Check sheet for the modelled part. Datum: model origin and axes. Units: mm. Give positions to 0.01 mm unless a question says otherwise; leave off trailing zeros.
from build123d import *

# Parameters (mm, degrees)
SKETCH1_W                      = 1219.2
SKETCH1_H                      = 1219.2
BOSS_EXTRUDE1_DEPTH            = 3.175
F_5_16_0_3125_DIAMETER_HOLE1_D = 7.9375
SKETCH5_W                      = 460.375
SKETCH5_H                      = 34.925
CUT_EXTRUDE1_DEPTH             = 863.110434124
CUT_EXTRUDE2_DEPTH             = 863.110434124
SKETCH8_W                      = 50.8
SKETCH8_H                      = 9.525
CUT_EXTRUDE3_DEPTH             = 863.110434124
SKETCH9_W                      = 298.45
SKETCH9_H                      = 3.175
CUT_EXTRUDE4_DEPTH             = 863.110434124
FILLET1_R                      = 3.175


with BuildPart() as part:
    # Sketch1 → Boss-Extrude1 (new body)
    with BuildSketch(Plane(origin=(0, 0, 0), x_dir=(1, 0, 0), z_dir=(0, 1, 0))):
        Rectangle(SKETCH1_W, SKETCH1_H)
    extrude(amount=BOSS_EXTRUDE1_DEPTH)

    # 5/16 (0.3125) Diameter Hole1 (through all)
    with Locations(Plane(origin=(0, 3.175, 0), x_dir=(1, 0, 0), z_dir=(0, 1, 0))):
        with Locations((-409.575, 377.825), (-22.225, 304.8), (22.225, 304.8), (409.575, 377.825), (-22.225, -304.8), (-409.575, -377.825), (409.575, -377.825), (22.225, -304.8)):
            Hole(F_5_16_0_3125_DIAMETER_HOLE1_D / 2)

    # Sketch5 → Cut-Extrude1 (cut, through all)
    with BuildSketch(Plane(origin=(0, 3.175, 0), x_dir=(1, 0, 0), z_dir=(0, 1, 0))):
        with Locations((-379.4125, 592.1375)):
            Rectangle(SKETCH5_W, SKETCH5_H)
        with Locations((379.4125, 592.1375)):
            Rectangle(SKETCH5_W, SKETCH5_H)
        with Locations((379.4125, -592.1375)):
            Rectangle(SKETCH5_W, SKETCH5_H)
        with Locations((-379.4125, -592.1375)):
            Rectangle(SKETCH5_W, SKETCH5_H)
    extrude(amount=-CUT_EXTRUDE1_DEPTH, mode=Mode.SUBTRACT)

    # Sketch7 → Cut-Extrude2 (cut, through all)
    with BuildSketch(Plane(origin=(0, 3.175, 0), x_dir=(1, 0, 0), z_dir=(0, 1, 0))):
        with BuildLine():
            Line((-428.625, 571.5), (-390.525, 571.5))
            ThreePointArc((-390.525, 571.5), (-384.175, 565.15), (-390.525, 558.8))
            Line((-390.525, 558.8), (-428.625, 558.8))
            ThreePointArc((-428.625, 558.8), (-434.975, 565.15), (-428.625, 571.5))
        make_face()
        with BuildLine():
            Line((-428.625, 196.85), (-390.525, 196.85))
            ThreePointArc((-390.525, 196.85), (-384.175, 190.5), (-390.525, 184.15))
            Line((-390.525, 184.15), (-428.625, 184.15))
            ThreePointArc((-428.625, 184.15), (-434.975, 190.5), (-428.625, 196.85))
        make_face()
        with BuildLine():
            Line((-38.1, 190.5), (-38.1, 152.4))
            ThreePointArc((-38.1, 152.4), (-44.45, 146.05), (-50.8, 152.4))
            Line((-50.8, 152.4), (-50.8, 190.5))
            ThreePointArc((-50.8, 190.5), (-44.45, 196.85), (-38.1, 190.5))
        make_face()
        with BuildLine():
            Line((-428.625, -571.5), (-390.525, -571.5))
            ThreePointArc((-390.525, -571.5), (-384.175, -565.15), (-390.525, -558.8))
            Line((-390.525, -558.8), (-428.625, -558.8))
            ThreePointArc((-428.625, -558.8), (-434.975, -565.15), (-428.625, -571.5))
        make_face()
        with BuildLine():
            Line((-428.625, -196.85), (-390.525, -196.85))
            ThreePointArc((-390.525, -196.85), (-384.175, -190.5), (-390.525, -184.15))
            Line((-390.525, -184.15), (-428.625, -184.15))
            ThreePointArc((-428.625, -184.15), (-434.975, -190.5), (-428.625, -196.85))
        make_face()
        with BuildLine():
            Line((-38.1, -190.5), (-38.1, -152.4))
            ThreePointArc((-38.1, -152.4), (-44.45, -146.05), (-50.8, -152.4))
            Line((-50.8, -152.4), (-50.8, -190.5))
            ThreePointArc((-50.8, -190.5), (-44.45, -196.85), (-38.1, -190.5))
        make_face()
        with BuildLine():
            Line((428.625, 571.5), (390.525, 571.5))
            ThreePointArc((390.525, 571.5), (384.175, 565.15), (390.525, 558.8))
            Line((390.525, 558.8), (428.625, 558.8))
            ThreePointArc((428.625, 558.8), (434.975, 565.15), (428.625, 571.5))
        make_face()
        with BuildLine():
            Line((428.625, 196.85), (390.525, 196.85))
            ThreePointArc((390.525, 196.85), (384.175, 190.5), (390.525, 184.15))
            Line((390.525, 184.15), (428.625, 184.15))
            ThreePointArc((428.625, 184.15), (434.975, 190.5), (428.625, 196.85))
        make_face()
        with BuildLine():
            Line((-44.45, 571.5), (44.45, 571.5))
            ThreePointArc((44.45, 571.5), (50.8, 565.15), (44.45, 558.8))
            Line((44.45, 558.8), (-44.45, 558.8))
            ThreePointArc((-44.45, 558.8), (-50.8, 565.15), (-44.45, 571.5))
        make_face()
        with BuildLine():
            Line((38.1, 190.5), (38.1, 152.4))
            ThreePointArc((38.1, 152.4), (44.45, 146.05), (50.8, 152.4))
            Line((50.8, 152.4), (50.8, 190.5))
            ThreePointArc((50.8, 190.5), (44.45, 196.85), (38.1, 190.5))
        make_face()
        with BuildLine():
            Line((428.625, -571.5), (390.525, -571.5))
            ThreePointArc((390.525, -571.5), (384.175, -565.15), (390.525, -558.8))
            Line((390.525, -558.8), (428.625, -558.8))
            ThreePointArc((428.625, -558.8), (434.975, -565.15), (428.625, -571.5))
        make_face()
        with BuildLine():
            Line((428.625, -196.85), (390.525, -196.85))
            ThreePointArc((390.525, -196.85), (384.175, -190.5), (390.525, -184.15))
            Line((390.525, -184.15), (428.625, -184.15))
            ThreePointArc((428.625, -184.15), (434.975, -190.5), (428.625, -196.85))
        make_face()
        with BuildLine():
            Line((38.1, -190.5), (38.1, -152.4))
            ThreePointArc((38.1, -152.4), (44.45, -146.05), (50.8, -152.4))
            Line((50.8, -152.4), (50.8, -190.5))
            ThreePointArc((50.8, -190.5), (44.45, -196.85), (38.1, -190.5))
        make_face()
        with BuildLine():
            Line((-44.45, -558.8), (44.45, -558.8))
            ThreePointArc((44.45, -558.8), (50.8, -565.15), (44.45, -571.5))
            Line((44.45, -571.5), (-44.45, -571.5))
            ThreePointArc((-44.45, -571.5), (-50.8, -565.15), (-44.45, -558.8))
        make_face()
    extrude(amount=-CUT_EXTRUDE2_DEPTH, mode=Mode.SUBTRACT)

    # Sketch8 → Cut-Extrude3 (cut, through all)
    with BuildSketch(Plane(origin=(0, 3.175, 0), x_dir=(1, 0, 0), z_dir=(0, 1, 0))):
        with Locations((-409.575, -569.9125)):
            Rectangle(SKETCH8_W, SKETCH8_H)
        with Locations((409.575, -569.9125)):
            Rectangle(SKETCH8_W, SKETCH8_H)
        with Locations((409.575, 569.9125)):
            Rectangle(SKETCH8_W, SKETCH8_H)
        with Locations((-409.575, 569.9125)):
            Rectangle(SKETCH8_W, SKETCH8_H)
    extrude(amount=-CUT_EXTRUDE3_DEPTH, mode=Mode.SUBTRACT)

    # Sketch9 → Cut-Extrude4 (cut, through all)
    with BuildSketch(Plane.XZ):
        with Locations((0, 608.0125)):
            Rectangle(SKETCH9_W, SKETCH9_H)
        with Locations((0, -608.0125)):
            Rectangle(SKETCH9_W, SKETCH9_H)
    extrude(amount=-CUT_EXTRUDE4_DEPTH, mode=Mode.SUBTRACT)

    # Fillet1
    fillet1_edges = [part.edges().sort_by_distance(p)[0] for p in [
        (-434.975, 1.5875, -574.675),
        (-384.175, 1.5875, -574.675),
        (434.975, 1.5875, -574.675),
        (384.175, 1.5875, -574.675),
        (434.975, 1.5875, 574.675),
        (384.175, 1.5875, 574.675),
        (-434.975, 1.5875, 574.675),
        (-384.175, 1.5875, 574.675),
        (-149.225, 1.5875, 606.425),
        (149.225, 1.5875, 606.425),
        (-149.225, 1.5875, -606.425),
        (149.225, 1.5875, -606.425),
        (-609.6, 1.5875, 574.675),
        (-149.225, 1.5875, 574.675),
        (149.225, 1.5875, 574.675),
        (609.6, 1.5875, 574.675),
        (609.6, 1.5875, -574.675),
        (149.225, 1.5875, -574.675),
        (-149.225, 1.5875, -574.675),
        (-609.6, 1.5875, -574.675),
    ]]
    fillet(fillet1_edges, radius=FILLET1_R)


solid = part.part
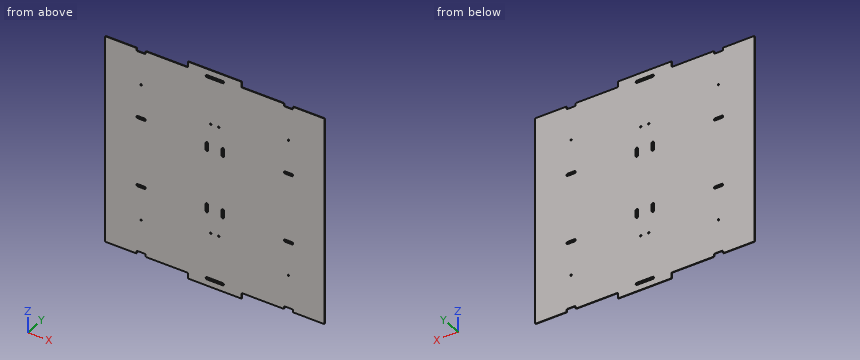
1) Gauge pin test, flat ends, axial feed: pin 1 (1.6 mm diameter, centred on x = -400, y = 2, fed in from +Z); pin 2 (1 mm diameter, centred on x = 543, y = 2, fed in from -Z) (3 decimals). Record the tip position at first contact, or that the pin passes through.
2) Sectioned sample at A-A on y = 2.55. Give the number of separate pieces and of enclosed holes in the cut face, then the cut area to 3 significant figures.
3) Scan lines: L1, parallel to X at y = 2.4, z = -171.5; L2, parallel to Z at x = -47, y = 1.6 (1 decimal); L3, parallel to Z at x = 180, y = 2 (3 decimals). Record each from-to range of solid material in increasing order.
Answers below:
1. pin 1: stops at z = 558.8
1. pin 2: stops at z = -574.675
2. separate pieces: 1
2. enclosed holes: 18
2. area: 1,410,000 mm2
3. L1: x = -609.6 to -50.8, -38.1 to 38.1, 50.8 to 609.6
3. L2: z = -606.4 to -571, -559.3 to -196.3, -146.6 to 146.6, 196.3 to 559.3, 571 to 606.4
3. L3: z = -574.675 to 574.675
